Input: dimensioned drawing with shaded views. Units: mm. Origin: part minimum x, y, z. Give positions to 0.01 mm unless a question says otherwise; leave off trailing zeros. Order: outer loops, then holes, each group sorted by start corner. A loop starts at its lowest first (then second) coordinate and runs counter-clockwise, first axis right, second up. Notation, with made-up numbers: (-1.5, -20) -> (16.5, -20) arc R26 ccw to (16.5, 2) -> close; hole circle Ø5 at (47, -26). An arc over 180 degrees is marked (long way). One line per question, with ' | ' between items. Start each with the question number.
(1) Section B-B (y = 4.75). Return loops of the section in (x, z).
(2) Mould query, pull axis X, two halves, no side actions, for the marked faces 1 and 2. Classes: +X half, -X half, draft (parallel to the pull), parting line (faces both ways), or undercut.
(3) First-contact query: pin 1 Ø1.5 at (y, z) = (5, 11.5) entering from +X; pin 2 Ø4 at (x, y) = (44.5, 2) entering from +Z. Flat tips, straight axial feed; report the tip coordinate or a pass-through.
(4) Ray query, L1, parallel to X at y = 6.25, z = 5.5; L2, parallel to Y at x = 37.5, z = 1.5; L3, parallel to Y at x = 71.5, z = 6.75. Return the intervals inside material, ascending.
(5) Section C-C (z = 6.5). Return loops of the section in (x, y).
(6) Section A-A (x = 3.5). Return loops of the section in (y, z), then the cut area to 3 significant figures.
(7) Section D-D (x = 37.5). Return loops of the section in (y, z).
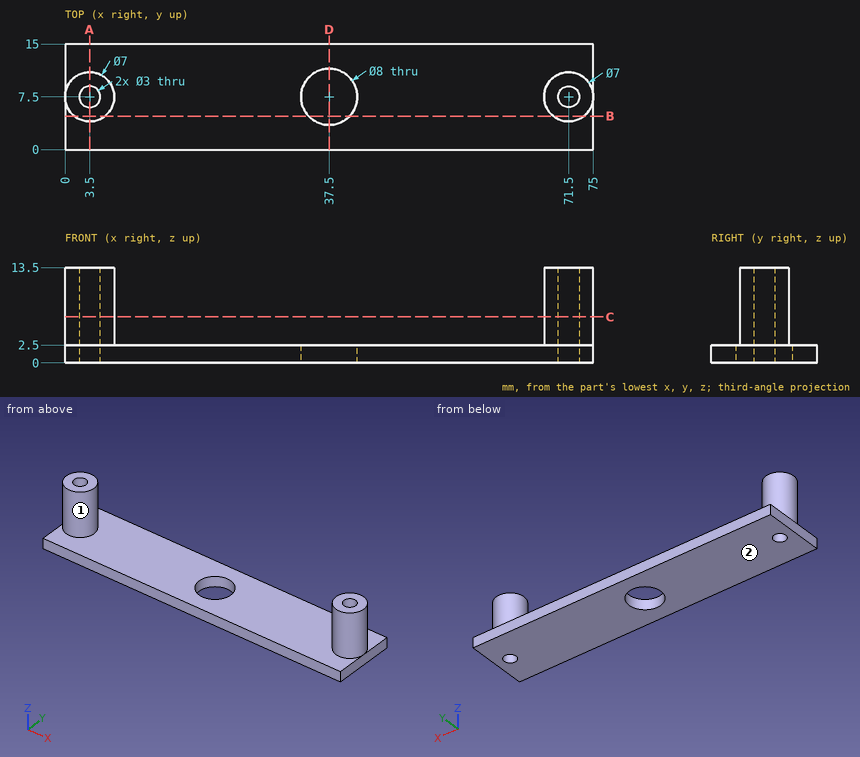
Response:
1) outline: (0, 0) -> (34.6, 0) -> (34.6, 2.5) -> (5.67, 2.5) -> (5.67, 13.5) -> (1.33, 13.5) -> (1.33, 2.5) -> (0, 2.5) -> close; (40.4, 0) -> (75, 0) -> (75, 2.5) -> (73.67, 2.5) -> (73.67, 13.5) -> (69.33, 13.5) -> (69.33, 2.5) -> (40.4, 2.5) -> close
2) face 1: undercut | face 2: draft
3) pin 1: stops at x = 74.53 | pin 2: stops at z = 2.5
4) L1: x = 0.23 to 2.67, 4.33 to 6.77, 68.23 to 70.67, 72.33 to 74.77 | L2: y = 0 to 3.5, 11.5 to 15 | L3: y = 4 to 6, 9 to 11
5) outline: circle Ø7 at (3.5, 7.5); circle Ø7 at (71.5, 7.5); hole circle Ø3 at (3.5, 7.5); hole circle Ø3 at (71.5, 7.5)
6) outline: (0, 0) -> (6, 0) -> (6, 13.5) -> (4, 13.5) -> (4, 2.5) -> (0, 2.5) -> close; (9, 0) -> (15, 0) -> (15, 2.5) -> (11, 2.5) -> (11, 13.5) -> (9, 13.5) -> close | area: 74.0 mm^2
7) outline: (0, 0) -> (3.5, 0) -> (3.5, 2.5) -> (0, 2.5) -> close; (11.5, 0) -> (15, 0) -> (15, 2.5) -> (11.5, 2.5) -> close
